The model under review builds one solid part; all positions refer to its coordinate system, in mm. A direction names the side the tool comes from. Give positions to 0.01 mm unless a question says otherwise; leave off trailing zeros. Loops run counter-clockwise (first coordinate to the right, second up) from the corner with the lowest first, then second, coordinate; pieces in that order, holes last. Notation, with made-up numbers: (20.25, -1) - (47.25, -1) arc R29 ccw to (47.25, 22) - close; hole circle Ø1 at (57.25, 64). An arc over 180 degrees is marked (long way). Return JSON: item names as keys, results as strings. Group by question number.
from build123d import *

# Parameters (mm, degrees)
SKETCH1_W           = 38.1
SKETCH1_H           = 6.35
BOSS_EXTRUDE1_DEPTH = 6.35
SKETCH2_R           = 2.4003
CUT_EXTRUDE1_DEPTH  = 8.89
FILLET1_R           = 0.635
SKETCH3_R           = 0.889
CUT_EXTRUDE2_DEPTH  = 3.81


with BuildPart() as part:
    # Sketch1 → Boss-Extrude1 (new body)
    with BuildSketch(Plane(origin=(0, 0, 0), x_dir=(1, 0, 0), z_dir=(0, 1, 0))):
        with Locations((19.05, 3.175)):
            Rectangle(SKETCH1_W, SKETCH1_H)
    extrude(amount=BOSS_EXTRUDE1_DEPTH)

    # Sketch2 → Cut-Extrude1 (cut)
    with BuildSketch(Plane.ZY):
        with Locations((-3.175, 3.175)):
            Circle(SKETCH2_R)
    extrude(amount=-CUT_EXTRUDE1_DEPTH, mode=Mode.SUBTRACT)

    # Fillet1
    fillet1_edges = [part.edges().sort_by_distance(p)[0] for p in [
        (0, 3.175, -6.35),
        (38.1, 3.175, -6.35),
        (38.1, 3.175, 0),
        (0, 3.175, 0),
    ]]
    fillet(fillet1_edges, radius=FILLET1_R)

    # Sketch3 → Cut-Extrude2 (cut)
    with BuildSketch(Plane.XZ):
        with Locations(Location((11.43, -3.175, 0), (0, 0, 270))):
            Circle(SKETCH3_R)
        with Locations(Location((26.67, -3.175, 0), (0, 0, 270))):
            Circle(SKETCH3_R)
    extrude(amount=-CUT_EXTRUDE2_DEPTH, mode=Mode.SUBTRACT)


solid = part.part
Item 1: Mouldability with a two-part tool opening along X and no side actions: class faces 1 (the face through (11, 3.81, -3)), 2 (the face through (0, 1.7, -0.9)), 3 (the face through (19, 0, -3)) as +X half, -X half, draft (parallel to the pull), parting line (faces both ways), or undercut.
Item 2: Take a section at C-C (y = 4.25). State the section outline as (x, z) points (3 decimals).
Item 3: For P1, Ø2.5, axis at x = 26.67, z = -3.175, coming from the -Y side; P2, Ø0.5, axis at x = 27, z = -3, coming from the -Y side, all flat-tipped, find the tip position at first contact; note any pin that passes through.
Item 4: Take a section at D-D (z = -1.75). State the section outline as (x, y) points, then the cut area to 3 significant figures.
Item 5: Take a section at B-B (y = 2.75). State the section outline as (x, z) points (3 decimals).
Item 6: Take a section at A-A (x = 26.67). State the section outline as (y, z) points.
Item 7: For L1, parallel to X at y = 2.25, z = -2.5; L2, parallel to X at y = 3.25, z = -2.75; L3, parallel to Z at x = 8.5, y = 2.75, list the stretches that pass through material, from the lowest coordinate up. Write a range as from..to.
Item 8: Tool access review of faces 4 (the face through (38.1, 3, -3)), 5 (the face through (8.89, 3, -3)), 6 (the face through (27, 3.81, -3)): name each direction out of +Z, -Z, +X, -X, +Y, -Y from which nothing blocks a thin tool from reaching the whole face with its end or side.
Check sheet entries:
{
 "1": {"face 1": "undercut", "face 2": "-X half", "face 3": "draft"},
 "2": {"outline": "(0, -5.715) arc R0.635 ccw to (0.635, -6.35) - (37.465, -6.35) arc R0.635 ccw to (38.1, -5.715) - (38.1, -0.635) arc R0.635 ccw to (37.465, 0) - (0.635, 0) arc R0.635 ccw to (0, -0.635) - (0, -1.029) - (8.89, -1.029) - (8.89, -5.321) - (0, -5.321) - close"},
 "3": {"P1": "stops at y = 0", "P2": "stops at y = 3.81"},
 "4": {"outline": "(0, 0) - (38.1, 0) - (38.1, 6.35) - (0, 6.35) - (0, 5.11) - (8.89, 5.11) - (8.89, 1.24) - (0, 1.24) - close", "area": "208 mm^2"},
 "5": {"outline": "(0, -5.715) arc R0.635 ccw to (0.635, -6.35) - (37.465, -6.35) arc R0.635 ccw to (38.1, -5.715) - (38.1, -0.635) arc R0.635 ccw to (37.465, 0) - (0.635, 0) arc R0.635 ccw to (0, -0.635) - (0, -0.813) - (8.89, -0.813) - (8.89, -5.537) - (0, -5.537) - close; hole circle Ø1.778 at (11.43, -3.175); hole circle Ø1.778 at (26.67, -3.175)"},
 "6": {"outline": "(0, -6.35) - (6.35, -6.35) - (6.35, 0) - (0, 0) - (0, -2.29) - (3.81, -2.29) - (3.81, -4.06) - (0, -4.06) - close"},
 "7": {"L1": "x = 8.89..10.85, 12.01..26.09, 27.25..38.1", "L2": "x = 8.89..10.65, 12.21..25.89, 27.45..38.1", "L3": "z = -6.35..-5.54, -0.81..0"},
 "8": {"face 4": "+Z, -Z, +X, +Y, -Y", "face 5": "-X", "face 6": "-Y"}
}
